Could you check a few things on this drawing? It's one solid part, dimensions in mm from its lowest x, y, z. A direction names the side the tool comes from. Give positions to 0.01 mm unless a question says otherwise; leave off trailing zeros. Write each loop counter-clockwise with the first axis right and the second up, starting at its lowest first coordinate (ties: lowest second). Pieces come first, ordered by that corner, then holes. Notation, with made-up numbers: M 9.25,80 L 52.25,80 A18 ccw 52.25,88 Z; hole C -29,26.5 d2. An arc over 180 degrees is marked long. Answer as CSV lines item,"result". Start each with the question number.
Q1. Suppose I cut it at B-B (x = 15). Write out the boundary of the cut face in (y, z) (3 decimals), then the cut area to 3 significant figures.
Q2. For pin 1 (2 mm diameter, centred on y = 9.5, z = 6, fed in from +X); pin 2 (2 mm diameter, centred on x = 5.5, z = 5, fed in from -Y); pin 3 (12 mm diameter, centred on x = 16, y = 38, fed in from +Z), each with a flat end and sliding along its axis, tell me the tip position at first contact or that it passes through.
Q3. Suppose I cut it at C-C (z = 6.5). Write out the boundary of the cut face in (x, y) (3 decimals).
Q4. If I drill on line 1 along X through (y, z) = (23, 4), over which ranges is the centre line in solid material (lowest first)?
Q5. Suppose I cut it at A-A (y = 31). Write out the boundary of the cut face in (x, z), then the cut area to 3 significant figures.
Q6. On a 3-axis mill with a long thin cutter (end or side, diameter ignored), from which of +Z, -Z, +X, -X, +Y, -Y can I reach the whole of each face in a straight line? I mean the marked faces 1 and 2. Say none if no direction works.
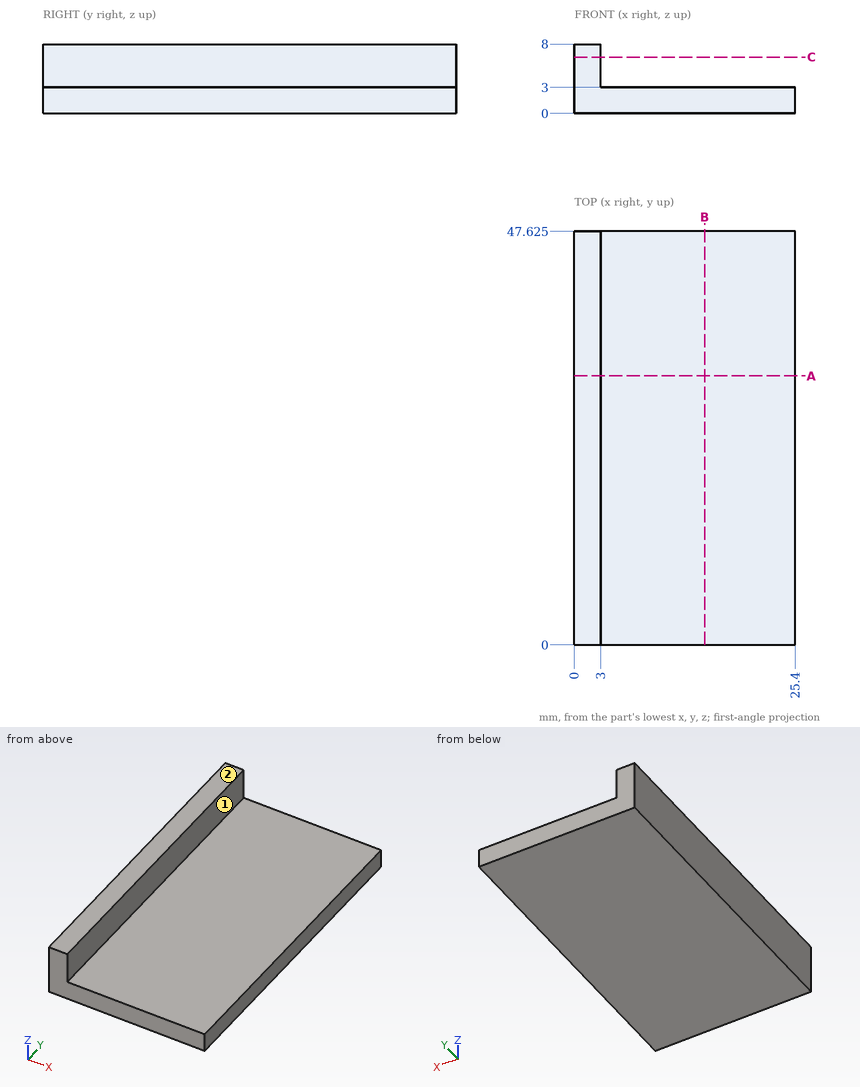
Resolved:
1,outline,"M 0,0 L 47.625,0 L 47.625,3 L 0,3 Z"
1,area,"143 mm^2"
2,pin 1,"x = 3"
2,pin 2,"through"
2,pin 3,"z = 3"
3,outline,"M 0,0 L 3,0 L 3,47.625 L 0,47.625 Z"
4,line 1,"0 to 3"
5,outline,"M 0,0 L 25.4,0 L 25.4,3 L 3,3 L 3,8 L 0,8 Z"
5,area,"91.2 mm^2"
6,face 1,"+Z, +X, +Y, -Y"
6,face 2,"+Z, +X, -X, +Y, -Y"
